CAD build for the part. Positions are in the model's coordinates, mm. A direction names the side the tool comes from. Give positions to 0.01 mm unless a question says otherwise; leave off trailing zeros. Order: outer loops, then holes, each group sorted by start corner. A loop starts at its lowest first (then second) coordinate and runs counter-clockwise, first axis right, second up. Notation, with made-up numbers: M 73.25,-15.5 L 98.25,-15.5 A18 cw 98.25,13.5 Z; hole C 77.5,36 d9. An arc over 180 degrees is marked long. Put each result on its own line as item: value. Start each with the question number.
1) Tool access for faces 1 (the face through (3.5, 0, 0)), 2 (the face through (17, 33, 0)), 3 (the face through (30.93, -30.85, 1.52)): list every direction of +Z, -Z, +X, -X, +Y, -Y with a clear straight run to the whole face (end or side of a thin tool).
2) Cut at A-A (z = 1). Write the cut outline in (x, y), and give its area (3 significant figures).
3) Pin check, flat tips, straight feed: pin 1 (3 mm diameter, centred on y = 9, z = -1, fed in from +X); pin 2 (7.5 mm diameter, centred on x = 13, y = 31, fed in from -Z); pin 3 (2.5 mm diameter, centred on x = 29, y = -32.75, fed in from -Z). Stop position of each tip, or through.
4) Drill centre lines: line 1 (Y direction, x = 29, z = 2); line 2 (X direction, y = -32.75, z = 1.35); line 3 (Y direction, x = 12.5, z = 0.5). Where is each one in solid material? Low to high. Write a range as [from, to].
5) Two-plate mould, pull along X, no slides. Class faces 4 (the face through (27.99, -31.64, 1.48)), 5 (the face through (17, -32, 0)), 6 (the face through (27.99, 33.86, 1.48)), 7 (the face through (4.1, 29.68, 1.52)): released by +X, released by -X, zero draft, split by the parting line, or undercut.
6) Cut at B-B (x = 19.5). Write the cut outline in (y, z).
7) Cut at C-C (y = -16.5). Write the cut outline in (x, z).
Autodesk Inventor part; units mm, degrees
ref_plane "YZ Plane" through (0, 0, 0) normal (1, 0, 0) x (0, 1, 0)
ref_plane "XZ Plane" through (0, 0, 0) normal (0, 1, 0) x (-1, 0, 0)
ref_plane "XY Plane" through (0, 0, 0) normal (0, 0, 1) x (1, 0, 0)
sketch "Sketch1" plane through (0, 0, 0) normal (0, 0, 1) x (1, 0, 0)
  line L0 (31.5, 30.25) -> (31.5, 35.25)
  line L1 (31.5, 35.25) -> (-3.5, 35.25)
  line L2 (-3.5, 35.25) -> (-3.5, 0)
  line L3 (-3.5, 0) -> (3.5, 0)
  line L4 (3.5, 0) -> (3.5, 30.25)
  line L5 (3.5, 30.25) -> (31.5, 30.25)
  point P0 (0, 0)
  point P1 (0, 0)
  point P2 (31.5, 32.75)
  dimension "d0" = 7
  dimension "d2" = 5
  dimension "d3" = 35
  dimension "d4" = 32.75
extrude "Extrusion1" add sketch "Sketch1" along normal blind 3
mirror "Mirror1" about plane through (0, 0, 0) normal (0, 1, 0) of "Extrusion1"
sketch "Sketch2" plane through (0, 0, 0) normal (0, 0, -1) x (-1, 0, 0)
  line L0 (-31.5, -35.25) -> (3.5, -35.25)
  line L1 (-31.5, 35.25) -> (3.5, 35.25)
  line L2 (3.5, -35.25) -> (-3.5, -35.25)
  line L3 (-3.5, -35.25) -> (-3.5, 35.25)
  line L4 (-3.5, 35.25) -> (3.5, 35.25)
  line L5 (3.5, 35.25) -> (3.5, -35.25)
  line L6 (-3.5, 30.25) -> (-3.5, -30.25)
  point P0 (0, 0)
  point P1 (-3.5, 0)
  point P2 (3.5, 35.25)
  point P3 (-3.5, -35.25)
extrude "Extrusion2" add sketch "Sketch2" along normal blind 3.5
sketch "Sketch3" plane through (0, 0, 3) normal (0, 0, 1) x (1, 0, 0)
  line L0 (29, 32.75) -> (29, -32.75)
  line L1 (31.5, 30.25) -> (31.5, 35.25)
  point P0 (0, 0)
  point P1 (29, 0)
  dimension "d16" = 65.5
  dimension "d18" = 2.5
hole "Hole1" at (29, -32.75, 3) at (29, 32.75, 3) direction (0, 0, -1) diameter 3 end through all
fillet "Fillet1" radius 2 8 edges at (31.5, -35.25, 1.5) (31.5, -30.25, 1.5) (31.5, 30.25, 1.5) (31.5, 35.25, 1.5) (-3.5, -35.25, -0.25) (-3.5, 35.25, -0.25) (3.5, -30.25, 1.5) (3.5, 30.25, 1.5)
properties part number "Display_Hilder" material "PC/ABS Plastic"
Solution:
1. face 1: -Z, +X
1. face 2: -Z, +X, +Y, -Y
1. face 3: +Z, -Z, +X
2. outline: M -3.5,-33.25 A2 ccw -1.5,-35.25 L 29.5,-35.25 A2 ccw 31.5,-33.25 L 31.5,-32.25 A2 ccw 29.5,-30.25 L 5.5,-30.25 A2 cw 3.5,-28.25 L 3.5,28.25 A2 cw 5.5,30.25 L 29.5,30.25 A2 ccw 31.5,32.25 L 31.5,33.25 A2 ccw 29.5,35.25 L -1.5,35.25 A2 ccw -3.5,33.25 Z; hole C 29,-32.75 d3; hole C 29,32.75 d3
2. area: 756 mm²
3. pin 1: x = 3.5
3. pin 2: z = 0
3. pin 3: through
4. line 1: [-35.25, -34.25], [-31.25, -30.25], [30.25, 31.25], [34.25, 35.25]
4. line 2: [-3.5, 27.5], [30.5, 31.5]
4. line 3: [-35.25, -30.25], [30.25, 35.25]
5. face 4: undercut
5. face 5: zero draft
5. face 6: undercut
5. face 7: released by +X
6. outline: M -35.25,0 L -30.25,0 L -30.25,3 L -35.25,3 Z; M 30.25,0 L 35.25,0 L 35.25,3 L 30.25,3 Z
7. outline: M -3.5,-3.5 L 3.5,-3.5 L 3.5,3 L -3.5,3 Z
